```python
from build123d import *

# Parameters (mm, degrees)
F1_DEPTH = 2
F2_DEPTH = 20
F3_R     = 0.5
F4_R     = 0.5


with BuildPart() as f1:
    # F0 (on Top) → F1 (new body)
    with BuildSketch(Plane.XY):
        with BuildLine():
            ThreePointArc((25.901247, 4.7573), (25.315461, 6.171513), (23.901247, 6.7573))
            Line((23.901247, 6.7573), (-19.681736, 6.7573))
            ThreePointArc((-19.681736, 6.7573), (-20.573861, 6.547304), (-21.278643, 5.961413))
            ThreePointArc((-21.278643, 5.961413), (-24.359844, -3.2427), (-21.278643, -12.446813))
            ThreePointArc((-21.278643, -12.446813), (-20.573861, -13.032704), (-19.681736, -13.2427))
            Line((-19.681736, -13.2427), (23.901247, -13.2427))
            ThreePointArc((23.901247, -13.2427), (25.315461, -12.656914), (25.901247, -11.2427))
            Line((25.901247, -11.2427), (25.901247, 4.7573))
        make_face()
    extrude(amount=F1_DEPTH)

    # F0 (on Top) → F2 (join)
    with BuildSketch(Plane.XY):
        with BuildLine():
            Line((27.901247, -11.2427), (27.901247, 4.7573))
            ThreePointArc((27.901247, 4.7573), (26.729674, 7.585727), (23.901247, 8.7573))
            Line((23.901247, 8.7573), (-19.681736, 8.7573))
            ThreePointArc((-19.681736, 8.7573), (-21.465986, 8.337307), (-22.875549, 7.165527))
            ThreePointArc((-22.875549, 7.165527), (-26.359844, -3.2427), (-22.875549, -13.650927))
            ThreePointArc((-22.875549, -13.650927), (-21.465986, -14.822708), (-19.681736, -15.2427))
            Line((-19.681736, -15.2427), (23.901247, -15.2427))
            ThreePointArc((23.901247, -15.2427), (26.729674, -14.071127), (27.901247, -11.2427))
        make_face()
        with BuildLine():
            Line((-19.681736, 6.7573), (23.901247, 6.7573))
            ThreePointArc((23.901247, 6.7573), (25.315461, 6.171513), (25.901247, 4.7573))
            Line((25.901247, 4.7573), (25.901247, -11.2427))
            ThreePointArc((25.901247, -11.2427), (25.315461, -12.656914), (23.901247, -13.2427))
            Line((23.901247, -13.2427), (-19.681736, -13.2427))
            ThreePointArc((-19.681736, -13.2427), (-20.573861, -13.032704), (-21.278643, -12.446813))
            ThreePointArc((-21.278643, -12.446813), (-24.359844, -3.2427), (-21.278643, 5.961413))
            ThreePointArc((-21.278643, 5.961413), (-20.573861, 6.547304), (-19.681736, 6.7573))
        make_face(mode=Mode.SUBTRACT)
    extrude(amount=F2_DEPTH)

    # F3
    f3_edges = [f1.edges().sort_by_distance(p)[0] for p in [
        (2.109756, -15.2427, 0),
    ]]
    fillet(f3_edges, radius=F3_R)

    # F4
    f4_edges = [f1.edges().sort_by_distance(p)[0] for p in [
        (2.109756, -15.2427, 20),
    ]]
    fillet(f4_edges, radius=F4_R)


solid = f1.part
```
Could you check a few things on this model? Use its own coordinates, in mm. A direction names the side the tool comes from. Round coordinates to 2 decimals unless told otherwise and drop trailing zeros. Loops run counter-clockwise (first coordinate to the right, second up) from the corner with the lowest first, then second, coordinate; pieces in that order, holes last. Notation, with made-up numbers: (-15.75, -25) -> (19.25, -25) arc R25 cw to (19.25, -5) -> close; hole circle Ø6 at (20.5, -21.75). An arc over 180 degrees is marked (long way). Put each result on its own line as item: value.
Q1. Please list where these lines run through material, in increasing order: line 1 (Y direction, x = 8.5, z = 5); line 2 (Z direction, x = -11, y = 4.5); line 3 (X direction, y = -1.5, z = 11.25). Write a range as from..to.
Checks:
line 1: -15.24..-13.24, 6.76..8.76
line 2: 0..2
line 3: -26.27..-24.26, 25.9..27.9
Q2. Thinking about a two-plate mould opening in X: for faces 3 (the flat face through (2, 6.757, 11)), 4 (the flat face through (25.901, -3, 11)), 5 (the cylindrical face through (-21.49, -14.81, 9.87)), 6 (the flat face through (27.901, -3, 10)), which applies, pulls with the +X half, pulls with the -X half, needs draft (parallel to the pull), parting line crosses it, or undercut?
Checks:
face 3: undercut
face 4: undercut
face 5: pulls with the -X half
face 6: pulls with the +X half
Q3. I want a section at A-A on z = 15. Write out the boundary of the cut face in (x, y), and give its area (3 significant figures).
Checks:
outline: (-22.88, -13.65) arc R4 ccw to (-19.68, -15.24) -> (23.9, -15.24) arc R4 ccw to (27.9, -11.24) -> (27.9, 4.76) arc R4 ccw to (23.9, 8.76) -> (-19.68, 8.76) arc R4 ccw to (-22.88, 7.17) arc R17.29 ccw to start; hole (-21.28, -12.45) arc R2 ccw to (-19.68, -13.24) -> (23.9, -13.24) arc R2 ccw to (25.9, -11.24) -> (25.9, 4.76) arc R2 ccw to (23.9, 6.76) -> (-19.68, 6.76) arc R2 ccw to (-21.28, 5.96) arc R15.29 ccw to start
area: 278 mm2
Q4. Which directions (+Z, -Z, +X, -X, +Y, -Y) give clear straight access to the entire face, cutting with the end or side of a thin tool? Please do faces 1 (the cylindrical face through (-20.59, 6.54, 10.87)), 2 (the cylindrical face through (26.761, 7.554, 9.867)).
Checks:
face 1: +Z
face 2: +Z, -Z, +X, +Y
Q5. I want a section at B-B on x = 18.5. Write out the boundary of the cut face in (y, z).
Checks:
outline: (-15.24, 0.5) arc R0.5 ccw to (-14.74, 0) -> (8.26, 0) arc R0.5 ccw to (8.76, 0.5) -> (8.76, 19.5) arc R0.5 ccw to (8.26, 20) -> (6.76, 20) -> (6.76, 2) -> (-13.24, 2) -> (-13.24, 20) -> (-14.74, 20) arc R0.5 ccw to (-15.24, 19.5) -> close
Q6. For pin 1 Ø6 at (x, y) = (12.5, -5.5) entering from +Z; pin 2 Ø2 at (y, z) = (3.5, 3.5) entering from -X, each with a flat end and sliding along its axis, tell me the tip position at first contact or that it passes through.
Checks:
pin 1: z = 2
pin 2: x = -25.38
